Can you work these out from the drawing? Everything is in mm from the part's minimum corner. A direction names the side the tool comes from. Coordinates: 2 decimals unless noted, no trailing zeros. Write each loop counter-clockwise with the first axis right and the second up, starting at its lowest first coordinate (ties: lowest second). Pieces come first, ordered by that corner, then holes.
(1) Imagine slicing it at C-C, the plane x = 76.5. List the corners of the cut face in (y, z) for me.
(2) Please list where these lines run through material, in increasing order: probe 1 along X at (y, z) = (13.5, 15.75); probe 2 along Y at (x, z) = (83.5, 20.25); probe 3 along Y at (x, z) = (82, 12.5).
(3) Which directions (+Z, -Z, +X, -X, +Y, -Y) give clear straight access to the entire face, cutting with the end or side of a thin tool? Please do the marked faces 1, 2 and 3.
(4) Imagine slicing it at B-B, the plane y = 13.75. List the corners of the cut face in (x, z) for me (3 decimals).
(5) Imagine slicing it at D-D, the plane x = 15. List the corners of the cut face in (y, z) for me.
(6) For pin 1 Ø4.5 at (x, y) = (1.5, 14.5) entering from +Z (3 decimals); pin 2 Ø3 at (x, z) = (96, 18.5) entering from -Y; pin 3 Ø10 at (x, z) = (78.5, 6.5) entering from +Y, each with a flat end and sliding along its axis, tell me the tip position at first contact or that it passes through.
(7) Imagine slicing it at A-A, the plane z = 13.75. List the corners of the cut face in (x, y) for me (3 decimals), plus the area to 3 significant figures.
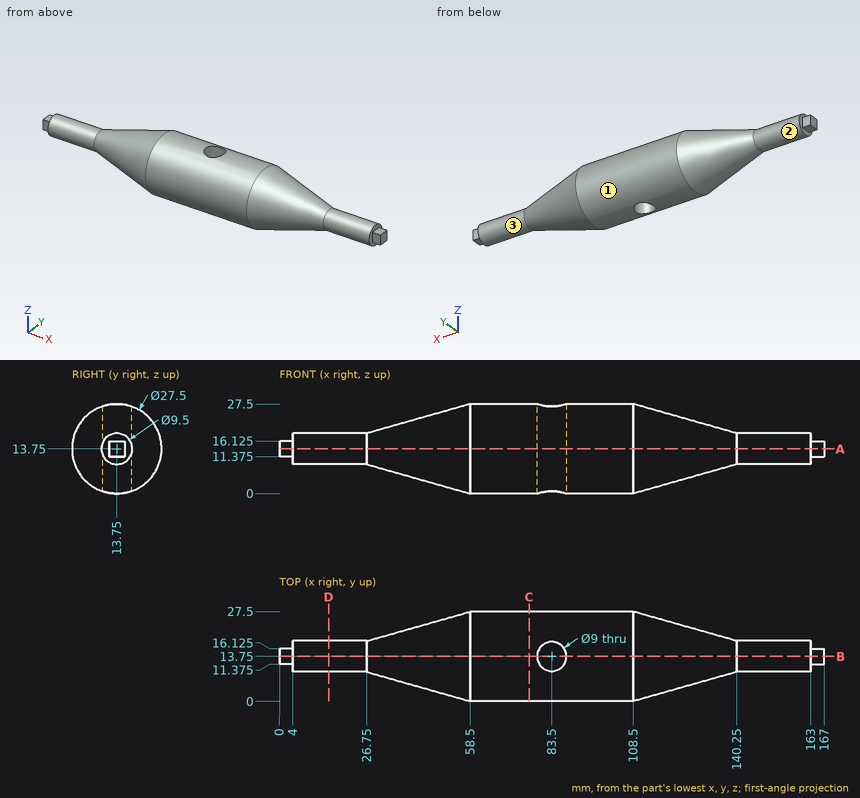
Recorded:
1. outline: circle Ø27.5 at (13.75, 13.75)
2. probe 1: x = 0 to 79.01, 87.99 to 167
2. probe 2: y = 1.63 to 9.25, 18.25 to 25.87
2. probe 3: y = 0.06 to 9.51, 17.99 to 27.44
3. face 1: +X, -X
3. face 2: -X
3. face 3: +X
4. outline: (0, 11.375) - (4, 11.375) - (4, 9) - (26.75, 9) - (58.5, 0) - (79, 0) - (79, 27.5) - (58.5, 27.5) - (26.75, 18.5) - (4, 18.5) - (4, 16.125) - (0, 16.125) - close; (88, 0) - (108.5, 0) - (140.25, 9) - (163, 9) - (163, 11.375) - (167, 11.375) - (167, 16.125) - (163, 16.125) - (163, 18.5) - (140.25, 18.5) - (108.5, 27.5) - (88, 27.5) - close
5. outline: circle Ø9.5 at (13.75, 13.75)
6. pin 1: stops at z = 16.125
6. pin 2: stops at y = 0.39
6. pin 3: stops at y = 27.31
7. outline: (0, 11.375) - (4, 11.375) - (4, 9) - (26.75, 9) - (58.5, 0) - (108.5, 0) - (140.25, 9) - (163, 9) - (163, 11.375) - (167, 11.375) - (167, 16.125) - (163, 16.125) - (163, 18.5) - (140.25, 18.5) - (108.5, 27.5) - (58.5, 27.5) - (26.75, 18.5) - (4, 18.5) - (4, 16.125) - (0, 16.125) - close; hole circle Ø9 at (83.5, 13.75)
7. area: 2,960 mm2
